Answer from the drawing. Dimensions are ordinates in mm from the lowest x, y and z of the part. A direction names the side the tool comes from. Give positions to 0.01 mm unless a question says otherwise; leave off trailing zeros. Order: outer loops, then holes, each group sorted by start corner. A loop starts at its lowest first (then second) coordinate and runs counter-clockwise, first axis right, second up.
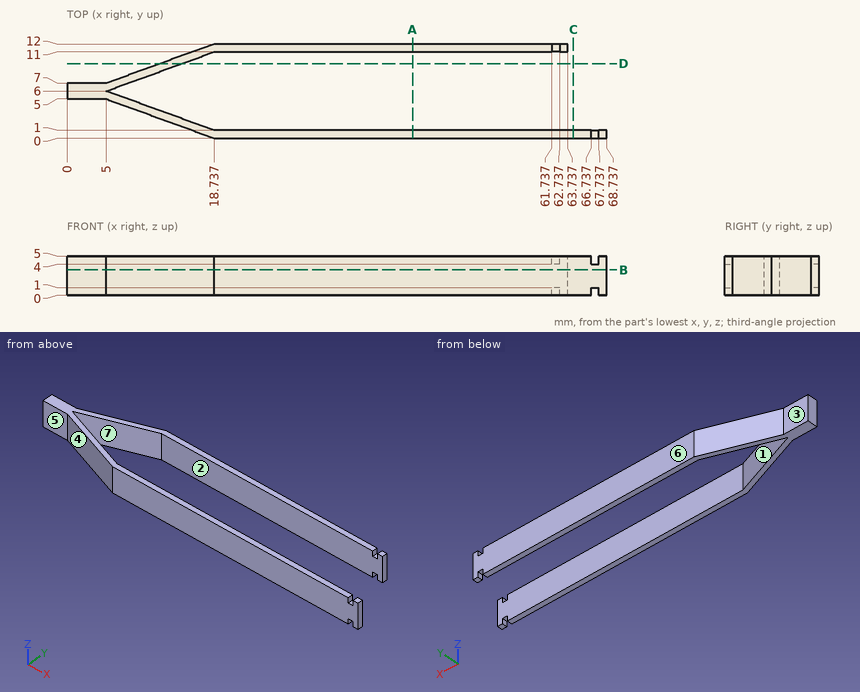
1. Given P1, Ø3, axis at x = 7.5, z = 3.5, coming from the +Y side; P2, Ø0.8, axis at y = 11.5, z = 3.5, coming from the +X side; P3, Ø1.5, axis at x = 2.5, z = 3.5, coming from the +Y side, each flat-ended and moving along its own axis, determine where each tip first touches the part or whether it passes through.
Findings below:
P1: stops at y = 8.46
P2: stops at x = 63.74
P3: stops at y = 7
2. The part is cut by section A-A (x = 44). Write down the section's boundary in (y, z).
Findings below:
outline: (0, 0) - (1, 0) - (1, 5) - (0, 5) - close; (11, 0) - (12, 0) - (12, 5) - (11, 5) - close
3. The part is cut by section D-D (y = 9.5). Write down the section's boundary in (x, z).
Findings below:
outline: (11.87, 0) - (14.62, 0) - (14.62, 5) - (11.87, 5) - close
4. Which of the six approach directions +Z, -Z, +X, -X, +Y, -Y give full straight-line access (tool end or side, diameter ignored) to the marked faces 5, 6 and 7?
Findings below:
face 5: +Z, -Z, -X, -Y
face 6: +Z, -Z, +X, -X, +Y
face 7: +Z, -Z, +X
5. The mould has two halves that part along Y. Classify the marked faces 1, 2, 3 and 4: pulls with the +Y half, pulls with the -Y half, needs draft (parallel to the pull), parting line crosses it, or undercut.
Findings below:
face 1: undercut
face 2: undercut
face 3: pulls with the +Y half
face 4: pulls with the -Y half
6. The part is cut by section B-B (z = 3.25). Write down the section's boundary in (x, y).
Findings below:
outline: (0, 5) - (5, 5) - (18.74, 0) - (68.74, 0) - (68.74, 1) - (18.74, 1) - (5, 6) - (18.74, 11) - (63.74, 11) - (63.74, 12) - (18.74, 12) - (5, 7) - (0, 7) - close
7. Straight lines are drawn through the part: probe 1 along Y at (x, z) = (21.5, 2.65); probe 2 along Y at (x, z) = (17, 0.8). For each, find the intervals that lie inside material, in ascending order.
Findings below:
probe 1: y = 0 to 1, 11 to 12
probe 2: y = 0.63 to 1.63, 10.37 to 11.37
8. The part is cut by section C-C (x = 64.5). Write down the section's boundary in (y, z).
Findings below:
outline: (0, 0) - (1, 0) - (1, 5) - (0, 5) - close
